Source: CAD feature listing. Evaluate the final solid. Frame: model axes, mm. Coordinates: 2 decimals unless noted, no trailing zeros. Order: outer loops, then holes, each group sorted by start corner. A loop starts at its lowest first (then second) coordinate and runs counter-clockwise, first axis right, second up.
Item 1: Section C-C on z = 4.5. State how many separate pieces and enclosed holes the cut face has, then the cut area to 3 significant figures.
Item 2: Section A-A on x = 85. Return the cut outline in (y, z), then the cut area to 3 significant figures.
Item 3: Section D-D on y = 27. Return the cut outline in (x, z), then the cut area to 4 significant figures.
Item 4: Section B-B on y = 2.25. Return the cut outline in (x, z), then the cut area to 3 significant figures.
Item 5: Ray query, line 1 (Y direction, x = 85, z = 4.75); line 2 (X direction, y = 3, z = 4.75); line 3 (X direction, y = 0, z = 9.5). Return the intervals inside material, ascending.
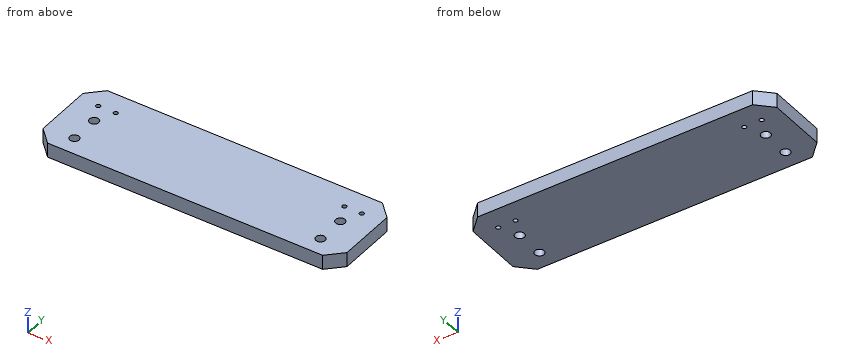
from build123d import *

# Parameters (mm, degrees)
SKETCH1_W           = 210
SKETCH1_H           = 60.5
SKETCH1_R           = 3.2
SKETCH1_R_2         = 1.5
BOSS_EXTRUDE1_DEPTH = 10
CHAMFER1_SIZE       = 10
CHAMFER2_SIZE       = 10


with BuildPart() as part:
    # Sketch1 → Boss-Extrude1 (new body)
    with BuildSketch(Plane.XY):
        Rectangle(SKETCH1_W, SKETCH1_H)
        with Locations((-85, 2.25)):
            Circle(SKETCH1_R, mode=Mode.SUBTRACT)
        with Locations((-85, -17.75)):
            Circle(SKETCH1_R, mode=Mode.SUBTRACT)
        with Locations((85, -17.75)):
            Circle(SKETCH1_R, mode=Mode.SUBTRACT)
        with Locations((85, 2.25)):
            Circle(SKETCH1_R, mode=Mode.SUBTRACT)
        with Locations((-91, 15.25)):
            Circle(SKETCH1_R_2, mode=Mode.SUBTRACT)
        with Locations((-79, 15.25)):
            Circle(SKETCH1_R_2, mode=Mode.SUBTRACT)
        with Locations((79, 15.25)):
            Circle(SKETCH1_R_2, mode=Mode.SUBTRACT)
        with Locations((91, 15.25)):
            Circle(SKETCH1_R_2, mode=Mode.SUBTRACT)
    extrude(amount=BOSS_EXTRUDE1_DEPTH)

    # Chamfer1
    chamfer1_edges = [part.edges().sort_by_distance(p)[0] for p in [
        (-105, 30.25, 5),
        (105, 30.25, 5),
    ]]
    chamfer(chamfer1_edges, length=CHAMFER1_SIZE)

    # Chamfer2
    chamfer2_edges = [part.edges().sort_by_distance(p)[0] for p in [
        (105, -30.25, 5),
        (-105, -30.25, 5),
    ]]
    chamfer(chamfer2_edges, length=CHAMFER2_SIZE)


solid = part.part
Answer list:
1. separate pieces: 1
1. enclosed holes: 8
1. area: 12,300 mm2
2. outline: (-30.25, 0) - (-20.95, 0) - (-20.95, 10) - (-30.25, 10) - close; (-14.55, 0) - (-0.95, 0) - (-0.95, 10) - (-14.55, 10) - close; (5.45, 0) - (30.25, 0) - (30.25, 10) - (5.45, 10) - close
2. area: 477 mm2
3. outline: (-98.25, 0) - (98.25, 0) - (98.25, 10) - (-98.25, 10) - close
3. area: 1,965 mm2
4. outline: (-105, 0) - (-88.2, 0) - (-88.2, 10) - (-105, 10) - close; (-81.8, 0) - (81.8, 0) - (81.8, 10) - (-81.8, 10) - close; (88.2, 0) - (105, 0) - (105, 10) - (88.2, 10) - close
4. area: 1,970 mm2
5. line 1: y = -30.25 to -20.95, -14.55 to -0.95, 5.45 to 30.25
5. line 2: x = -105 to -88.11, -81.89 to 81.89, 88.11 to 105
5. line 3: x = -105 to -87.28, -82.72 to 82.72, 87.28 to 105
